Source: CAD feature listing. Evaluate the final solid. Frame: model axes, mm. Coordinates: 2 decimals unless noted, no trailing zeros. Order: outer loops, then holes, each group sorted by start corner. A loop starts at its lowest first (then second) coordinate and runs counter-clockwise, first axis right, second up. Notation, with made-up numbers: (71.25, 25.25) -> (76.25, 25.25) arc R22 ccw to (76.25, 56.25) -> close; hole circle Ø10 at (-29.5, -9). An arc over 180 degrees is marked (long way). Put each result on its own line as item: value.
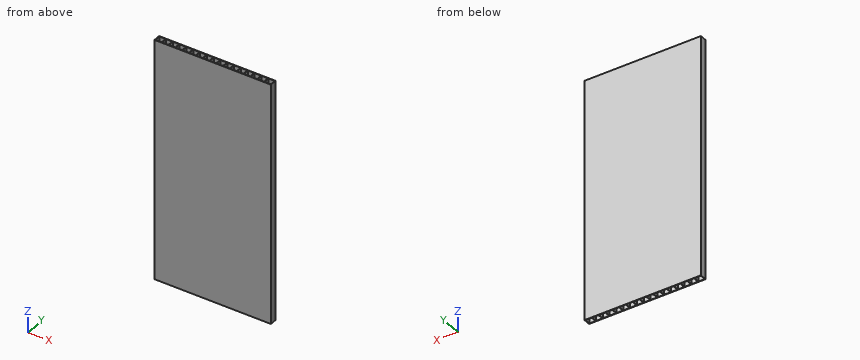
Autodesk Inventor part; units mm, degrees
ref_plane "YZ Plane" through (0, 0, 0) normal (1, 0, 0) x (0, 1, 0)
ref_plane "XZ Plane" through (0, 0, 0) normal (0, 1, 0) x (-1, 0, 0)
ref_plane "XY Plane" through (0, 0, 0) normal (0, 0, 1) x (1, 0, 0)
sketch "Sketch1" plane through (0, 0, 0) normal (0, 0, 1) x (1, 0, 0)
  line L0 (0, 0) -> (108.458, 0)
  line L1 (108.458, 0) -> (108.458, 6.35)
  line L2 (108.458, 6.35) -> (0, 6.35)
  line L3 (0, 6.35) -> (0, 0)
  line L4 (0.508, 0.5094) -> (6.35, 0.5094)
  line L5 (6.35, 0.5094) -> (6.35, 5.842)
  line L6 (6.35, 5.842) -> (0.508, 5.842)
  line L7 (0.508, 5.842) -> (0.508, 0.5094)
  line L8 (6.858, 0.5094) -> (12.7, 0.5094)
  line L9 (12.7, 0.5094) -> (12.7, 5.842)
  line L10 (12.7, 5.842) -> (6.858, 5.842)
  line L11 (6.858, 5.842) -> (6.858, 0.5094)
  line L12 (13.208, 0.5094) -> (19.05, 0.5094)
  line L13 (19.05, 0.5094) -> (19.05, 5.842)
  line L14 (19.05, 5.842) -> (13.208, 5.842)
  line L15 (13.208, 5.842) -> (13.208, 0.5094)
  line L16 (19.558, 0.5094) -> (25.4, 0.5094)
  line L17 (25.4, 0.5094) -> (25.4, 5.842)
  line L18 (25.4, 5.842) -> (19.558, 5.842)
  line L19 (19.558, 5.842) -> (19.558, 0.5094)
  line L20 (25.908, 0.5094) -> (31.75, 0.5094)
  line L21 (31.75, 0.5094) -> (31.75, 5.842)
  line L22 (31.75, 5.842) -> (25.908, 5.842)
  line L23 (25.908, 5.842) -> (25.908, 0.5094)
  line L24 (32.258, 0.5094) -> (38.1, 0.5094)
  line L25 (38.1, 0.5094) -> (38.1, 5.842)
  line L26 (38.1, 5.842) -> (32.258, 5.842)
  line L27 (32.258, 5.842) -> (32.258, 0.5094)
  line L28 (38.608, 0.5094) -> (44.45, 0.5094)
  line L29 (44.45, 0.5094) -> (44.45, 5.842)
  line L30 (44.45, 5.842) -> (38.608, 5.842)
  line L31 (38.608, 5.842) -> (38.608, 0.5094)
  line L32 (44.958, 0.5094) -> (50.8, 0.5094)
  line L33 (50.8, 0.5094) -> (50.8, 5.842)
  line L34 (50.8, 5.842) -> (44.958, 5.842)
  line L35 (44.958, 5.842) -> (44.958, 0.5094)
  line L36 (51.308, 0.5094) -> (57.15, 0.5094)
  line L37 (57.15, 0.5094) -> (57.15, 5.842)
  line L38 (57.15, 5.842) -> (51.308, 5.842)
  line L39 (51.308, 5.842) -> (51.308, 0.5094)
  line L40 (57.658, 0.5094) -> (63.5, 0.5094)
  line L41 (63.5, 0.5094) -> (63.5, 5.842)
  line L42 (63.5, 5.842) -> (57.658, 5.842)
  line L43 (57.658, 5.842) -> (57.658, 0.5094)
  line L44 (64.008, 0.5094) -> (69.85, 0.5094)
  line L45 (69.85, 0.5094) -> (69.85, 5.842)
  line L46 (69.85, 5.842) -> (64.008, 5.842)
  line L47 (64.008, 5.842) -> (64.008, 0.5094)
  line L48 (70.358, 0.5094) -> (76.2, 0.5094)
  line L49 (76.2, 0.5094) -> (76.2, 5.842)
  line L50 (76.2, 5.842) -> (70.358, 5.842)
  line L51 (70.358, 5.842) -> (70.358, 0.5094)
  line L52 (76.708, 0.5094) -> (82.55, 0.5094)
  line L53 (82.55, 0.5094) -> (82.55, 5.842)
  line L54 (82.55, 5.842) -> (76.708, 5.842)
  line L55 (76.708, 5.842) -> (76.708, 0.5094)
  line L56 (83.058, 0.5094) -> (88.9, 0.5094)
  line L57 (88.9, 0.5094) -> (88.9, 5.842)
  line L58 (88.9, 5.842) -> (83.058, 5.842)
  line L59 (83.058, 5.842) -> (83.058, 0.5094)
  line L60 (89.408, 0.5094) -> (95.25, 0.5094)
  line L61 (95.25, 0.5094) -> (95.25, 5.842)
  line L62 (95.25, 5.842) -> (89.408, 5.842)
  line L63 (89.408, 5.842) -> (89.408, 0.5094)
  line L64 (95.758, 0.5094) -> (101.6, 0.5094)
  line L65 (101.6, 0.5094) -> (101.6, 5.842)
  line L66 (101.6, 5.842) -> (95.758, 5.842)
  line L67 (95.758, 5.842) -> (95.758, 0.5094)
  line L68 (102.108, 0.5094) -> (107.95, 0.5094)
  line L69 (107.95, 0.5094) -> (107.95, 5.842)
  line L70 (107.95, 5.842) -> (102.108, 5.842)
  line L71 (102.108, 5.842) -> (102.108, 0.5094)
  dimension "d0" = 108.458
  dimension "d1" = 6.35
  dimension "d2" = 0.5094
  dimension "d3" = 0.508
  dimension "d4" = 0.508
  dimension "d5" = 5.842
  dimension "d8" = 6.35
extrude "Extrusion1" add sketch "Sketch1" along normal blind 225.425
properties part number "8 ball polycarb side"
1. Ray query, line 1 along Y through (x, z) = (27.5, 80). Return the intervals inside material, ascending.
Numbers:
line 1: y = 0 to 0.51, 5.84 to 6.35
2. Cut plane B-B on y = 3.5. Count the separate pieces of the cut face and the enclosed holes in it, plus the area to 3 significant figures.
Numbers:
separate pieces: 18
enclosed holes: 0
area: 2,060 mm2
3. First-contact query: pin 1 (1.5 mm diameter, centred on x = 34, y = 5, fed in from -Z). Flat tip, straight axial feed; report the tip coordinate or a pass-through.
Numbers:
pin 1: passes through
4. Cut plane A-A on x = 92.5. Output: boundary loops of the cut face in (y, z) (3 decimals), plus the area to 3 significant figures.
Numbers:
outline: (0, 0) -> (0.509, 0) -> (0.509, 225.425) -> (0, 225.425) -> close; (5.842, 0) -> (6.35, 0) -> (6.35, 225.425) -> (5.842, 225.425) -> close
area: 229 mm2
